Autodesk Inventor part; units mm, degrees
ref_plane "YZ Plane" through (0, 0, 0) normal (1, 0, 0) x (0, 1, 0)
ref_plane "XZ Plane" through (0, 0, 0) normal (0, 1, 0) x (-1, 0, 0)
ref_plane "XY Plane" through (0, 0, 0) normal (0, 0, 1) x (1, 0, 0)
sketch "Sketch1" plane through (0, 0, 0) normal (0, 0, 1) x (1, 0, 0)
  line L0 (-105.4358, -42.0697) -> (85.0642, -42.0697)
  line L1 (85.0642, -42.0697) -> (85.0642, 186.5303)
  line L2 (85.0642, 186.5303) -> (-105.4358, 186.5303)
  line L3 (-105.4358, 186.5303) -> (-105.4358, -42.0697)
  line L4 (-105.4358, -42.0697) -> (-156.2358, -42.0697)
  line L5 (-156.2358, -42.0697) -> (-156.2358, 237.3303)
  line L6 (-156.2358, 237.3303) -> (135.8642, 237.3303)
  line L7 (135.8642, 237.3303) -> (135.8642, -42.0697)
  line L8 (135.8642, -42.0697) -> (85.0642, -42.0697)
  point P0 (0, 0)
  dimension "d0" = 228.6
  dimension "d1" = 190.5
  dimension "d2" = 50.8
  dimension "d3" = 279.4
  dimension "d4" = 292.1
extrude "Door Frame CR" add sketch "Sketch1" along normal mid plane 8.89 contours L4 L5 L6 L7 L8 L1 L2 L3
sketch "Sketch2" plane through (-156.2358, -42.0697, 4.445) normal (-1, 0, 0) x (0, 0, 1)
  line L0 (-8.89, 279.4) -> (-8.89, 0)
  line L1 (-8.89, 279.4) -> (0, 279.4)
  line L2 (0, 279.4) -> (0, 0)
  line L3 (0, 0) -> (-8.89, 0)
  line L4 (-8.89, 0) -> (-8.89, 279.4)
  point P0 (-4.445, 42.0697)
extrude "Door Frame left Extruded" add sketch "Sketch2" along normal blind 685.8
sketch "Sketch4" plane through (135.8642, -42.0697, 4.445) normal (1, 0, 0) x (0, 0, -1)
  line L0 (0, 0) -> (0, 279.4)
  line L1 (8.89, 228.6) -> (8.89, 0)
  line L2 (0, 279.4) -> (8.89, 279.4)
  line L3 (8.89, 279.4) -> (8.89, 0)
  line L4 (8.89, 0) -> (0, 0)
  line L5 (0, 0) -> (0, 279.4)
  point P0 (4.445, 42.0697)
extrude "Door Frame right Extruded" add sketch "Sketch4" along normal blind 685.8
sketch "Sketch5" plane through (0, 0, 4.445) normal (0, 0, 1) x (1, 0, 0)
  line L0 (-842.0358, 237.3303) -> (-842.0358, -42.0697)
  line L1 (821.6642, 237.3303) -> (821.6642, -42.0697)
  line L2 (-842.0358, -42.0697) -> (821.6642, -42.0697)
  line L3 (821.6642, -42.0697) -> (821.6642, -36.9897)
  line L4 (821.6642, -36.9897) -> (-842.0358, -36.9897)
  line L5 (-842.0358, -36.9897) -> (-842.0358, -42.0697)
  point P0 (0, 0)
  dimension "d11" = 5.08
extrude "Floor" add sketch "Sketch5" along normal blind 762
sketch "Sketch7" plane through (-105.4358, -36.9897, 4.445) normal (0, 1, 0) x (1, 0, 0)
  line L0 (-736.6, 0) -> (0, 0)
  line L1 (-736.6, -762) -> (927.1, -762)
  line L2 (-736.6, 0) -> (-723.9, 0)
  line L3 (-723.9, 0) -> (-723.9, -749.3)
  line L4 (-723.9, -762) -> (-736.6, -762)
  line L5 (-736.6, -762) -> (-736.6, 0)
  line L6 (927.1, 8.89) -> (927.1, -762)
  line L7 (-723.9, -762) -> (927.1, -762)
  line L8 (927.1, -762) -> (927.1, -749.3)
  line L9 (914.4, -749.3) -> (-723.9, -749.3)
  line L10 (190.5, 0) -> (927.1, 0)
  line L11 (914.4, -749.3) -> (914.4, 0)
  line L12 (914.4, 0) -> (927.1, 0)
  line L13 (927.1, 0) -> (927.1, -749.3)
  point P0 (105.4358, 4.445)
  dimension "d21" = 12.7
extrude "Walls" add sketch "Sketch7" along normal blind 274.6375
sketch "Door Frame" plane through (0, 0, 4.445) normal (0, 0, 1) x (1, 0, 0)
  line L0 (-105.4358, -36.9897) -> (-105.4358, 186.5303)
  line L1 (-105.4358, -36.9897) -> (-113.0558, -36.9897)
  line L2 (-113.0558, -36.9897) -> (-113.0558, 186.5303)
  line L3 (-105.4358, 186.5303) -> (-105.4358, -36.9897)
  line L4 (-105.4358, 186.5303) -> (85.0642, 186.5303)
  line L5 (92.6842, 185.3187) -> (92.6842, -36.9897)
  line L6 (92.6842, -36.9897) -> (85.0642, -36.9897)
  line L7 (85.0642, -36.9897) -> (85.0642, 186.5303)
  line L8 (-105.4358, 186.5303) -> (85.0642, 186.5303)
  line L9 (92.6842, 185.3187) -> (92.6842, 194.1503)
  line L10 (92.6842, 194.1503) -> (-113.0558, 194.1503)
  line L11 (-113.0558, 194.1503) -> (-113.0558, 186.5303)
  point P0 (0, 0)
  dimension "d27" = 7.62
  dimension "d28" = 7.62
  dimension "d29" = 7.62
extrude "Extrusion7" add sketch "Door Frame" along normal blind 7.9375
fillet "Dorr Fillet" radius 0.508 1 edges at (-113.0558, 194.1503, 8.4138)
fillet "Door Fillet" radius 0.508 1 edges at (92.6842, 194.1503, 8.4138)
sketch "Sketch9" plane through (0, 0, 4.445) normal (0, 0, -1) x (-1, 0, 0)
  line L0 (-85.0642, -36.9897) -> (-85.0642, -42.0697)
  line L1 (-85.0642, -36.9897) -> (105.4358, -36.9897)
  line L2 (105.4358, -36.9897) -> (105.4358, -42.0697)
  line L3 (105.4358, -42.0697) -> (-85.0642, -42.0697)
  line L4 (-85.0642, -42.0697) -> (-85.0642, -36.9897)
  point P0 (0, 0)
extrude "Door floor" add sketch "Sketch9" along normal blind 8.89
sketch "Sketch13" plane through (808.9642, -36.9897, 753.745) normal (0, 0, -1) x (-1, 0, 0)
  line L0 (-12.7, -5.08) -> (-12.7, 274.6375)
  line L1 (-12.7, 31.9391) -> (1651, 31.9391)
  line L2 (1651, 31.9391) -> (1651, -1.0809)
  line L3 (1651, -1.0809) -> (-12.7, -1.0809)
  line L4 (-12.7, -1.0809) -> (-12.7, 31.9391)
  point P0 (808.9642, 36.9897)
  dimension "d36" = 33.02
extrude "wall board" add sketch "Sketch13" along normal blind 2.54
sketch "Sketch14" plane through (808.9642, -36.9897, 4.445) normal (-1, 0, 0) x (0, 0, 1)
  line L0 (-8.89, -5.08) -> (-8.89, 274.32)
  line L1 (762, -5.08) -> (762, 274.6375)
  line L2 (-8.89, -5.08) -> (762, -5.08)
  line L3 (762, -5.08) -> (762, 27.94)
  line L4 (762, 27.94) -> (-8.89, 27.94)
  line L5 (-8.89, 27.94) -> (-8.89, -5.08)
  point P0 (-4.445, 36.9897)
  dimension "d39" = 33.02
properties part number "Top Office Layer (safety save)"
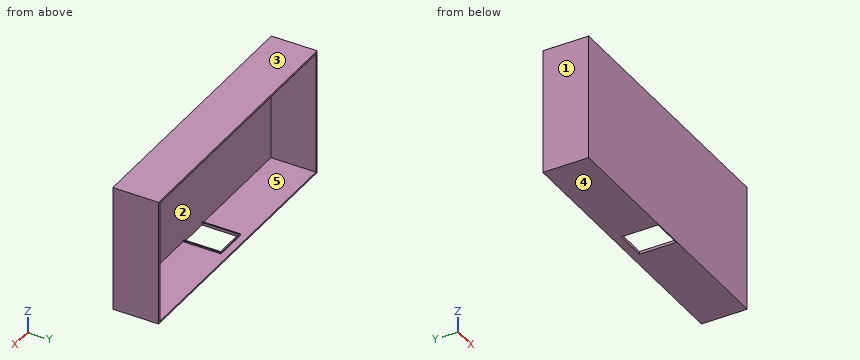
The listing builds one solid part. Answer for the finished solid, in the listing's coordinates (mm). Face numbers are marked on the shaded views. A direction names the side the tool comes from. Round coordinates to 2 decimals unless told otherwise and drop trailing zeros. Loops run counter-clockwise (first coordinate to the right, second up) from the corner with the lowest first, then second, coordinate; pieces in that order, holes last. Notation, with made-up numbers: (-12.75, 29) - (34.25, 29) arc R8 cw to (34.25, 42) - close; hole circle Ø11 at (-5.75, 30.25). An arc over 180 degrees is marked (long way). Return JSON: item names as keys, results as strings. Group by question number.
1. The part is cut by section D-D on x = -441. Determine the outline of the cut face in (y, z) (3 decimals), then the cut area to 3 significant figures.
2. The part is cut by section C-C on z = 324. Determine the outline of the cut face in (x, y), then the cut area to 3 significant figures.
3. The part is cut by section B-B on y = 52.5. Determine the outline of the cut face in (x, z) (1 decimal).
4. Each of these flat-tipped pins is pushed along its axis until it touches: P1, Ø12, axis at x = -541.5, z = 485, coming from the +Y side; P2, Ø8.5, axis at x = 15.5, z = 8.5, coming from the +Y side; P3, Ø3, axis at x = 9, y = 3.5, coming from the -Z side (3 decimals). Where does it stop, or does it pass through?
5. The part is cut by section A-A on x = 26. Determine the outline of the cut face in (y, z) (1 decimal), then the cut area to 3 significant figures.
6. Which of the six approach directions +Z, -Z, +X, -X, +Y, -Y give full straight-line access (tool end or side, diameter ignored) to the marked faces 4 and 5?
7. Consider probe 1 along Z at (x, y) = (-151.5, -30) (3 decimals); probe 2 along X at (y, z) = (149.5, 710); probe 3 along Z at (x, y) = (339, 79.5) (3 decimals). Determine where each line is inside the solid, lowest interval first.
8. The mould has two halves that part along X. Classify the marked faces 1, 2 and 3: pulls with the +X half, pulls with the -X half, needs draft (parallel to the pull), parting line crosses it, or undercut.
Resolved:
{
 "1": {"outline": "(-42.07, -4.445) - (237.33, -4.445) - (237.33, 4.445) - (-36.99, 4.445) - (-36.99, 751.205) - (-5.051, 751.205) - (-5.051, 753.745) - (237.648, 753.745) - (237.648, 766.445) - (-42.07, 766.445) - close", "area": "9,920 mm²"},
 "2": {"outline": "(-842.04, -42.07) - (821.66, -42.07) - (821.66, 237.65) - (808.96, 237.65) - (808.96, -36.99) - (-829.34, -36.99) - (-829.34, 237.65) - (-842.04, 237.65) - close", "area": "15,400 mm²"},
 "3": {"outline": "(-842, -4.4) - (-105.4, -4.4) - (-105.4, 12.4) - (-113.1, 12.4) - (-113.1, 4.4) - (-829.3, 4.4) - (-829.3, 753.7) - (809, 753.7) - (809, 4.4) - (92.7, 4.4) - (92.7, 12.4) - (85.1, 12.4) - (85.1, -4.4) - (821.7, -4.4) - (821.7, 766.4) - (-842, 766.4) - close"},
 "4": {"P1": "stops at y = -36.99", "P2": "stops at y = 237.33", "P3": "stops at z = 753.745"},
 "5": {"outline": "(-42.1, -4.4) - (-37, -4.4) - (-37, 751.2) - (-5.1, 751.2) - (-5.1, 753.7) - (237.6, 753.7) - (237.6, 766.4) - (-42.1, 766.4) - close; (186.5, -4.4) - (237.3, -4.4) - (237.3, 4.4) - (194.2, 4.4) - (194.2, 12.4) - (186.5, 12.4) - close", "area": "8,000 mm²"},
 "6": {"face 4": "-Z, +X, -X, +Y, -Y", "face 5": "+Y"},
 "7": {"probe 1": "z = -4.445 to 4.445, 751.205 to 766.445", "probe 2": "x = -842.04 to -829.34, 808.96 to 821.66", "probe 3": "z = -4.445 to 4.445, 753.745 to 766.445"},
 "8": {"face 1": "pulls with the -X half", "face 2": "undercut", "face 3": "needs draft"}
}
